Solid Edge part; units mm, degrees
revolve "RevolvedProtrusion1" [suppressed]
fillet "Round1" [suppressed]
revolve "RevolvedProtrusion2" [suppressed]
revolve "RevolvedProtrusion3" [suppressed]
sketch "Sketch1" plane through (0, 0, 0) normal (0, -1, 0) x (1, 0, 0)
  line L0 (9, 15) -> (9, -15)
  line L1 (9, -15) -> (7.2, -15)
  line L2 (7.2, -15) -> (6.65, -14.5)
  line L3 (6.65, -14.5) -> (6.65, -9.9)
  line L4 (6.65, -9.9) -> (6.05, -9.9)
  line L5 (5, -7.9) -> (6.05, -9.9)
  line L6 (5, -7.9) -> (5, 7.9)
  line L7 (6.05, 9.9) -> (5, 7.9)
  line L8 (6.05, 9.9) -> (6.65, 9.9)
  line L9 (6.65, 9.9) -> (6.65, 14.5)
  line L10 (6.65, 14.5) -> (7.2, 15)
  line L11 (7.2, 15) -> (9, 15)
  dimension "D1" = 6.65
  dimension "D2" = 9
  dimension "D3" = 9
revolve "RevolvedProtrusion4" add sketch "Sketch1" angle 360 about axis through (0, 0, 54) along (0, 0, -1)
Part model, mm, in its own coordinate system. A direction names the side the tool comes from. Coordinates: 2 decimals unless noted, no trailing zeros. Loops run counter-clockwise (first coordinate to the right, second up) from the corner with the lowest first, then second, coordinate; pieces in that order, holes last. Notation, with made-up numbers: (39, 72) - (96, 72) arc R17 cw to (96, 95) - close; hole circle Ø11 at (48.25, 0). An arc over 180 degrees is marked (long way). Write each question's results on one line, items separated by ' | '. Start each with the question number.
Q1. Which spindle directions (+Z, -Z, +X, -X, +Y, -Y) get a long thin tool onto all of the face, cutting with end or side? Do faces 1 (the flat face through (-2, 6, -9.9)), 2 (the cylindrical face through (3.07, -5.9, 12.23)), 3 (the cylindrical face through (-1.08, -4.88, 0.11)). Say none if no direction does.
Q2. Drop flat-ended pins along their axis: pin 1 Ø3 at (x, y) = (3.5, 2.5) entering from +Z; pin 2 Ø1 at (x, y) = (-2, 5.5) entering from +Z; pin 3 Ø1 at (x, z) = (-6.5, 11.5) entering from -Y. Give the stop position or say it passes through.
Q3. Two-plate mould, pull along X, no slides. Class faces 4 (the cylindrical face through (-1.172, -8.923, -0.21)), 5 (the flat face through (3, -7, -15)), 6 (the cylindrical face through (3.07, -5.9, -12.17)): +X half, -X half, draft (parallel to the pull), parting line (faces both ways), or undercut.
Q4. Slice it at D-D on z = 9.5. Give the cut face in (x, y), and give its area (3 significant figures).
Q5. Slice it at C-C on z = -1.5. Give the cut face in (x, y), and give its area (3 significant figures).
Q6. Probe line 1 along X through (y, z) = (0, -12.85); line 2 along X through (y, z) = (0, 0.5). List the from-to ranges inside material, lowest first.
Q7. Slice it at A-A on x = 0. Give the cut face in (y, z), and give its area (3 significant figures).
Answer:
1) face 1: -Z | face 2: +Z | face 3: +Z, -Z
2) pin 1: stops at z = 9.43 | pin 2: stops at z = 9.9 | pin 3: stops at y = -6.71
3) face 4: parting line | face 5: draft | face 6: undercut
4) outline: circle Ø18 at (0, 0); hole circle Ø11.68 at (0, 0) | area: 147 mm2
5) outline: circle Ø18 at (0, 0); hole circle Ø10 at (0, 0) | area: 176 mm2
6) line 1: x = -9 to -6.65, 6.65 to 9 | line 2: x = -9 to -5, 5 to 9
7) outline: (-9, -15) - (-7.2, -15) - (-6.65, -14.5) - (-6.65, -9.9) - (-6.05, -9.9) - (-5, -7.9) - (-5, 7.9) - (-6.05, 9.9) - (-6.65, 9.9) - (-6.65, 14.5) - (-7.2, 15) - (-9, 15) - close; (5, -7.9) - (6.05, -9.9) - (6.65, -9.9) - (6.65, -14.5) - (7.2, -15) - (9, -15) - (9, 15) - (7.2, 15) - (6.65, 14.5) - (6.65, 9.9) - (6.05, 9.9) - (5, 7.9) - close | area: 202 mm2
